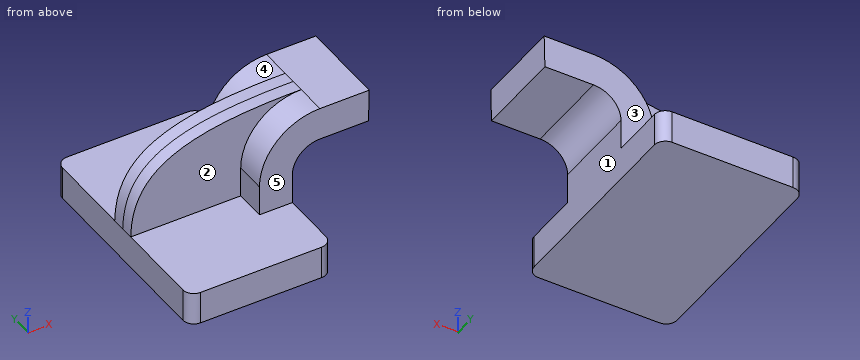
from build123d import *

# Parameters (mm, degrees)
F1_DEPTH = 63.5
F2_DEPTH = 25.4
F3_DEPTH = 7.62
F4_R     = 6.35


with BuildPart() as f1:
    # F0 (on Front) → F1 (new body, symmetric)
    with BuildSketch(Plane.XZ):
        Polygon((-41.275, -9.525), (41.275, -9.525), (41.275, 9.525), (22.225, 9.525), (-41.275, 9.525), align=None)
    extrude(amount=F1_DEPTH, both=True)

    # F0 (on Front) → F2 (join, symmetric)
    with BuildSketch(Plane.XZ):
        with BuildLine():
            Line((22.225, 9.525), (41.275, 9.525))
            Line((41.275, 9.525), (41.275, 27.0002))
            ThreePointArc((41.275, 27.0002), (45.92468, 38.22552), (57.15, 42.8752))
            Line((57.15, 42.8752), (60.325, 42.8752))
            Line((60.325, 42.8752), (60.325, 61.9252))
            Line((60.325, 61.9252), (57.15, 61.9252))
            ThreePointArc((57.15, 61.9252), (32.454296, 51.695904), (22.225, 27.0002))
            Line((22.225, 27.0002), (22.225, 9.525))
        make_face()
        Polygon((85.611328, 61.9252), (60.325, 61.9252), (60.325, 42.8752), (85.194737, 42.8752), align=None)
    extrude(amount=F2_DEPTH, both=True)

    # F0 (on Front) → F3 (join, symmetric)
    with BuildSketch(Plane.XZ):
        with BuildLine():
            add(Edge.make_bspline(
                [(-41.275, 9.525), (-40.618513, 46.65922), (-15.205906, 62.490027), (57.15, 61.9252)],
                knots=[0, 0, 0, 0, 111.504536, 111.504536, 111.504536, 111.504536], degree=3))
            Line((-41.275, 9.525), (22.225, 9.525))
            Line((22.225, 9.525), (22.225, 27.0002))
            ThreePointArc((22.225, 27.0002), (32.454296, 51.695904), (57.15, 61.9252))
        make_face()
    extrude(amount=F3_DEPTH, both=True)

    # F4
    f4_edges = [f1.edges().sort_by_distance(p)[0] for p in [
        (41.275, -63.5, 0),
        (41.275, 63.5, 0),
        (-41.275, -63.5, 0),
        (-41.275, 63.5, 0),
    ]]
    fillet(f4_edges, radius=F4_R)


solid = f1.part
Could you check a few things on this model? Use its own coordinates, in mm. Face numbers are marked on the shaded views. A direction names the side the tool comes from. Round coordinates to 2 decimals unless told otherwise and drop trailing zeros. Write each loop counter-clockwise with the first axis right and the second up, starting at its lowest first coordinate (ties: lowest second). Pieces come first, ordered by that corner, then holes. Notation, with made-up numbers: (-34.5, -14.75) - (5.5, -14.75) arc R15 cw to (5.5, -0.75) - close; hole circle Ø5 at (55, 74). An arc over 180 degrees is marked (long way). Put each result on its own line as item: value. Start each with the question number.
(1) I want a section at C-C, the plane x = 61. Please give me the cut outline in (y, z), plus the area to 3 significant figures.
(2) I need wall thicknesses on probe 1 along X at (y, z) = (22, 21) (3 decimals); probe 2 along Y at (x, z) = (-34, 23); probe 3 along Z at (x, y) = (-24, 13.5) (3 decimals). Which ranges of each line are inside material? Lowest first, please.
(3) I want a section at B-B, the plane y = -13. Please give me the cut outline in (x, z) (3 decimals), plus the area to 3 significant figures.
(4) I want a section at D-D, the plane y = 49. Please give me the cut outline in (x, z) (3 decimals), plus the area to 3 significant figures.
(5) For the marked faces 1, 2, 3, 4 and 5, which set-ups out of +Z, -Z, +X, -X, +Y, -Y let a thin tool reach every point of the face, with its end or its side?
(6) Will these pins go through, and if not, where does the flat tip stop? pin 1 (2 mm diameter, centred on x = 28, y = 44, fed in from +Z) (3 decimals); pin 2 (3 mm diameter, centred on x = -9, z = 23.5, fed in from +Y); pin 3 (14 mm diameter, centred on x = 75.5, y = -4, fed in from -Z).
(7) I want a section at A-A, the plane z = 4.5. Please give me the cut outline in (x, y) (3 decimals).
Here are the results:
1. outline: (-25.4, 42.88) - (25.4, 42.88) - (25.4, 61.93) - (-25.4, 61.93) - close
1. area: 968 mm^2
2. probe 1: x = 22.225 to 41.275
2. probe 2: y = -7.62 to 7.62
2. probe 3: z = -9.525 to 9.525
3. outline: (-41.275, -9.525) - (41.275, -9.525) - (41.275, 27) arc R15.875 cw to (57.15, 42.875) - (85.195, 42.875) - (85.611, 61.925) - (57.15, 61.925) arc R34.925 ccw to (22.225, 27) - (22.225, 9.525) - (-41.275, 9.525) - close
3. area: 3,200 mm^2
4. outline: (-41.275, -9.525) - (41.275, -9.525) - (41.275, 9.525) - (-41.275, 9.525) - close
4. area: 1,570 mm^2
5. face 1: -Z, +X, +Y, -Y
5. face 2: +Z, -X, -Y
5. face 3: +Z, +X, -X, +Y
5. face 4: +Z, -X, +Y
5. face 5: +Z, +X, -X, -Y
6. pin 1: stops at z = 9.525
6. pin 2: stops at y = 7.62
6. pin 3: stops at z = 42.88
7. outline: (-41.275, -57.15) arc R6.35 ccw to (-34.925, -63.5) - (34.925, -63.5) arc R6.35 ccw to (41.275, -57.15) - (41.275, 57.15) arc R6.35 ccw to (34.925, 63.5) - (-34.925, 63.5) arc R6.35 ccw to (-41.275, 57.15) - close
